```python
from build123d import *

# Parameters (mm, degrees)
SKETCH1_W           = 30
SKETCH1_H           = 12
BOSS_EXTRUDE1_DEPTH = 3
SKETCH3_W           = 5
SKETCH3_H           = 3
BOSS_EXTRUDE2_DEPTH = 3
SKETCH4_R           = 1.5
CUT_EXTRUDE1_DEPTH  = 10


with BuildPart() as part:
    # Sketch1 → Boss-Extrude1 (new body)
    with BuildSketch(Plane(origin=(0, 0, 0), x_dir=(0, 0, -1), z_dir=(1, 0, 0))):
        Rectangle(SKETCH1_W, SKETCH1_H)
    extrude(amount=BOSS_EXTRUDE1_DEPTH)

    # Sketch3 → Boss-Extrude2 (add)
    with BuildSketch(Plane(origin=(3, 0, 0), x_dir=(0, 0, -1), z_dir=(1, 0, 0))):
        with Locations((-10, 7.5)):
            Rectangle(SKETCH3_W, SKETCH3_H)
        with Locations((0, 7.5)):
            Rectangle(SKETCH3_W, SKETCH3_H)
        with Locations((10, 7.5)):
            Rectangle(SKETCH3_W, SKETCH3_H)
        with Locations((10, -7.5)):
            Rectangle(SKETCH3_W, SKETCH3_H)
        with Locations((0, -7.5)):
            Rectangle(SKETCH3_W, SKETCH3_H)
        with Locations((-10, -7.5)):
            Rectangle(SKETCH3_W, SKETCH3_H)
    extrude(amount=-BOSS_EXTRUDE2_DEPTH)

    # Sketch4 → Cut-Extrude1 (cut)
    with BuildSketch(Plane(origin=(3, 0, 0), x_dir=(0, 0, -1), z_dir=(1, 0, 0))):
        Circle(SKETCH4_R)
        with BuildLine():
            ThreePointArc((10.970300816, -3.45), (11.5, 0), (10.970300816, 3.45))
            ThreePointArc((10.970300816, 3.45), (9.089392014, 4.430908802), (8.108483212, 2.55))
            ThreePointArc((8.108483212, 2.55), (8.5, 0), (8.108483212, -2.55))
            ThreePointArc((8.108483212, -2.55), (9.089392014, -4.430908802), (10.970300816, -3.45))
        make_face()
    extrude(amount=-CUT_EXTRUDE1_DEPTH, mode=Mode.SUBTRACT)


solid = part.part
```
Design review of the part built by this model. Coordinates are the model's own, in mm. A direction names the side the tool comes from. Round coordinates to 2 decimals unless told otherwise and drop trailing zeros. Write each loop counter-clockwise with the first axis right and the second up, starting at its lowest first coordinate (ties: lowest second). Pieces come first, ordered by that corner, then holes. Notation, with made-up numbers: (-11, -9.75) -> (33, -9.75) arc R20 ccw to (33, 24.25) -> close; hole circle Ø1 at (63, 43). An arc over 180 degrees is marked (long way). Write item = value, one per line. Start each with the question number.
1) Take a section at A-A, the plane y = 0. State the section outline as (x, z) points, plus the area to 3 significant figures.
2) Clearance check with flat-ended pins moving along their axes: pin 1 (0.8 mm diameter, centred on x = 1, z = 13.5, fed in from +Y); pin 2 (1.5 mm diameter, centred on x = 1.5, z = 6, fed in from -Y); pin 3 (0.9 mm diameter, centred on x = 1.5, y = -7.5, fed in from +Z). State where each tip first meets the part, or that it passes through.
3) Take a section at B-B, the plane z = 0. State the section outline as (x, y) points.
4) Mouldability with a two-part tool opening along Y and no side actions: class faces 1 (the face through (1.52, 0.07, 1.5)), 2 (the face through (2, 7, 7.5)), 3 (the face through (1, 6, 5)) as +Y half, -Y half, draft (parallel to the pull), parting line (faces both ways), or undercut.
5) Tool access review of faces 4 (the face through (1, -6, -14)), 5 (the face through (1, 6, -5)), 6 (the face through (1, -6, -5)): name each direction out of +Z, -Z, +X, -X, +Y, -Y from which nothing blocks a thin tool from reaching the whole face with its end or side.
6) Wall thickness on probe 1 along Y at (x, z) = (0.75, 0); probe 2 along Y at (x, z) = (1.8, -4.25); probe 3 along Y at (x, z) = (1.2, 1): over which ranges is each line inside the solid? List them lowest first. Write a range as from..to.
7) Take a section at C-C, the plane x = 1.55. Count the separate pieces of the cut face and the enclosed holes in it, plus the area to 3 significant figures.
8) Take a section at D-D, the plane y = -3. State the section outline as (x, z) points.
Results list:
q1.outline = (0, -15) -> (3, -15) -> (3, -11.5) -> (0, -11.5) -> close; (0, -8.5) -> (3, -8.5) -> (3, -1.5) -> (0, -1.5) -> close; (0, 1.5) -> (3, 1.5) -> (3, 15) -> (0, 15) -> close
q1.area = 72.0 mm²
q2.pin_1 = 6
q2.pin_2 = -6
q2.pin_3 = 12.5
q3.outline = (0, -9) -> (3, -9) -> (3, -1.5) -> (0, -1.5) -> close; (0, 1.5) -> (3, 1.5) -> (3, 9) -> (0, 9) -> close
q4.face_1 = undercut
q4.face_2 = draft
q4.face_3 = +Y half
q5.face_4 = -Z, +X, -X, -Y
q5.face_5 = +X, -X, +Y
q5.face_6 = +X, -X, -Y
q6.probe_1 = -9..-1.5, 1.5..9
q6.probe_2 = -6..6
q6.probe_3 = -9..-1.12, 1.12..9
q7.separate_pieces = 1
q7.enclosed_holes = 2
q7.area = 418 mm²
q8.outline = (0, -15) -> (3, -15) -> (3, -11.1) -> (0, -11.1) -> close; (0, -8.04) -> (3, -8.04) -> (3, 15) -> (0, 15) -> close
